```python
from build123d import *

# Parameters (mm, degrees)
SKETCH026_R     = 2.5
PAD010_DEPTH    = 15
POCKET010_DEPTH = 4


with BuildPart() as part:
    # Sketch026 → Pad010 (new body)
    with BuildSketch(Plane.XY):
        with BuildLine():
            ThreePointArc((7.1470904861, 4.890715447), (6.25, 10.8253175473), (0.6619385767, 8.6349196476))
            ThreePointArc((-0.6619385767, 8.6349196476), (0, 7.9978308267), (0.6619385767, 8.6349196476))
            ThreePointArc((-0.6619385767, 8.6349196476), (-6.25, 10.8253175473), (-7.1470904861, 4.890715447))
            ThreePointArc((-7.8090290628, 3.7442042006), (-6.9263246711, 3.9989154133), (-7.1470904861, 4.890715447))
            ThreePointArc((-7.8090290628, 3.7442042006), (-12.5, 0), (-7.8090290628, -3.7442042006))
            ThreePointArc((-7.1470904861, -4.890715447), (-6.9263246711, -3.9989154133), (-7.8090290628, -3.7442042006))
            ThreePointArc((-7.1470904861, -4.890715447), (-6.25, -10.8253175473), (-0.6619385767, -8.6349196476))
            ThreePointArc((0.6619385767, -8.6349196476), (0, -7.9978308267), (-0.6619385767, -8.6349196476))
            ThreePointArc((0.6619385767, -8.6349196476), (6.25, -10.8253175473), (7.1470904861, -4.890715447))
            ThreePointArc((7.8090290628, -3.7442042006), (6.9263246711, -3.9989154133), (7.1470904861, -4.890715447))
            ThreePointArc((7.8090290628, -3.7442042006), (12.5, 0), (7.8090290628, 3.7442042006))
            ThreePointArc((7.1470904861, 4.890715447), (6.9263246711, 3.9989154133), (7.8090290628, 3.7442042006))
        make_face()
        Circle(SKETCH026_R, mode=Mode.SUBTRACT)
    extrude(amount=PAD010_DEPTH)

    # Sketch027 (on Face15 of Pad010) → Pocket010 (cut)
    with BuildSketch(Plane.XY.offset(15)):
        Polygon((2.225, -3.8538130468), (4.45, 0), (2.225, 3.8538130468), (-2.225, 3.8538130468), (-4.45, 0), (-2.225, -3.8538130468), align=None)
    extrude(amount=-POCKET010_DEPTH, mode=Mode.SUBTRACT)

    # Sketch028 → Groove001 (revolve, cut)
    with BuildSketch(Plane.XZ):
        with BuildLine():
            ThreePointArc((12.5, 10), (7.0833333333, 6.25), (5, 0))
            Line((5, 0), (13.5, 0))
            Line((13.5, 0), (13.5, 10))
            Line((13.5, 10), (12.5, 10))
        make_face()
    revolve(axis=Axis((0, 0, 0), (0, 0, 1)), mode=Mode.SUBTRACT)


solid = part.part
```
Geometry: final body of the model. Coordinates: model frame, mm. A direction names the side the tool comes from. Give positions to 0.01 mm unless a question says otherwise; leave off trailing zeros. Order: outer loops, then holes, each group sorted by start corner. A loop starts at its lowest first (then second) coordinate and runs counter-clockwise, first axis right, second up. Notation, with made-up numbers: (2.5, 26) -> (59.5, 26) arc R23 ccw to (59.5, 44) -> close; hole circle Ø6 at (86.5, 78.5). An arc over 180 degrees is marked (long way). Write each question's results on one line, items separated by ' | '. Start each with the question number.
1) Set-up query: faces 1 (the cylindrical face through (-12.5, 0.1, 12.2)), 2 (the flat face through (0, -3.854, 13)). Return all of +Z, -Z, +X, -X, +Y, -Y with unobstructed straight access to the full face (end or side cutting, diameter ignored); none if empty.
2) Draft query along Y for faces 3 (the flat face through (-3.322, 1.954, 13.028)), 4 (the flat face through (-3, 3, 15)), 5 (the cylindrical face through (0.014, -7.998, 11.094)), 6 (the flat face through (0, 3.854, 13)). Return one class per face: pulls with the +Y half, pulls with the -Y half, needs draft (parallel to the pull), parting line crosses it, or undercut.
3) Section B-B (z = 8.25). Return loops of the section in (x, y), then the cut area to 3 significant figures.
4) Line query: line 1 (X direction, y = 0, z = 2.75); line 2 (X direction, y = 0, z = 7.25); line 3 (Y direction, x = -2.25, z = 4.5). Output: solid intervals per line, ascending. Write a range as from..to.
5) Section A-A (x = 0). Return loops of the section in (y, z), then the cut area to 3 significant figures.
6) First-contact query: pin 1 (3 mm diameter, centred on x = 0, z = 12.5, fed in from +Y) (3 decimals); pin 2 (4.5 mm diameter, centred on x = 0, z = 12.5, fed in from -Y); pin 3 (1.5 mm diameter, centred on x = 6, z = 6.5, fed in from -Y). Flat tips, straight axial feed; report the tip coordinate or a pass-through.
7) Section D-D (x = -7.5). Count the separate pieces of the cut face and the enclosed holes in it, then the cut area to 3 significant figures.
Calculated:
1) face 1: +Z, -Z | face 2: +Z
2) face 3: undercut | face 4: needs draft | face 5: pulls with the -Y half | face 6: undercut
3) outline: (-8.21, -3.81) arc R3.84 ccw to (-7.81, -3.74) arc R0.66 cw to (-7.15, -4.89) arc R3.84 ccw to (-7.41, -5.21) arc R9.06 ccw to (-0.8, -9.02) arc R3.84 ccw to (-0.66, -8.63) arc R0.66 cw to (0.66, -8.63) arc R3.84 ccw to (0.8, -9.02) arc R9.06 ccw to (7.41, -5.21) arc R3.84 ccw to (7.15, -4.89) arc R0.66 cw to (7.81, -3.74) arc R3.84 ccw to (8.21, -3.81) arc R9.06 ccw to (8.21, 3.81) arc R3.84 ccw to (7.81, 3.74) arc R0.66 cw to (7.15, 4.89) arc R3.84 ccw to (7.41, 5.21) arc R9.06 ccw to (0.8, 9.02) arc R3.84 ccw to (0.66, 8.63) arc R0.66 cw to (-0.66, 8.63) arc R3.84 ccw to (-0.8, 9.02) arc R9.06 ccw to (-7.41, 5.21) arc R3.84 ccw to (-7.15, 4.89) arc R0.66 cw to (-7.81, 3.74) arc R3.84 ccw to (-8.21, 3.81) arc R9.06 ccw to start; hole circle Ø5 at (0, 0) | area: 231 mm2
4) line 1: -5.37..-2.5, 2.5..5.37 | line 2: -7.94..-2.5, 2.5..7.94 | line 3: -5.59..-1.09, 1.09..5.59
5) outline: (-8, 7.31) arc R10.42 cw to (-5, 0) -> (-2.5, 0) -> (-2.5, 11) -> (-3.85, 11) -> (-3.85, 15) -> (-8, 15) -> close; (2.5, 0) -> (5, 0) arc R10.42 cw to (8, 7.31) -> (8, 15) -> (3.85, 15) -> (3.85, 11) -> (2.5, 11) -> close | area: 124 mm2
6) pin 1: y = 10.095 | pin 2: y = -10.73 | pin 3: y = -5.47
7) separate pieces: 3 | enclosed holes: 0 | area: 108 mm2
